Geometry check sheet. Reference: drawing and pictorial views, mm from the part's lowest x, y, z. A direction names the side the tool comes from. Give positions to 0.01 mm unless a question says otherwise; leave off trailing zeros. Loops run counter-clockwise (first coordinate to the right, second up) from the corner with the lowest first, then second, coordinate; pieces in that order, holes last. Notation, with made-up numbers: (32, 34.25) -> (85, 34.25) arc R33 cw to (85, 62.25) -> close; hole circle Ø7 at (-2, 23.5). An arc over 180 degrees is marked (long way). One line per item, written item: value. Start each with the question number.
(1) Gauge pin test, flat ends, axial feed: pin 1 Ø1.4 at (x, y) = (6.39, 19.11) entering from +Z; pin 2 Ø2 at (x, y) = (12.75, 3.75) entering from -Z; pin 3 Ø1.5 at (x, z) = (17, 2.5) entering from +Y. Record the tip position at first contact, or that the pin passes through.
(2) Sectioned sample at A-A, the plane y = 12.75. Record the cut outline in (x, z).
(3) Scan lines: line 1 along X through (y, z) = (6, 5.15); line 2 along Y through (x, z) = (12.75, 4.5); line 3 along Z through (x, y) = (10.5, 24). Record each from-to range of solid material in increasing order. Write a range as from..to.
(4) Tool access check on the marked faces 1 and 2. Record the directions out of +Z, -Z, +X, -X, +Y, -Y that give a thin tool (end or side, any length) a straight path to the whole face; none if there is none.
(5) Draft check along Y on the marked faces 3, 4 and 5. Enter one of: pulls with the +Y half, pulls with the -Y half, needs draft (parallel to the pull), parting line crosses it, or undercut.
(6) Sectioned sample at D-D, the plane x = 3.75. Record the cut outline in (y, z).
(7) Sectioned sample at C-C, the plane z = 1.85. Record the cut outline in (x, y), then the cut area to 3 significant figures.
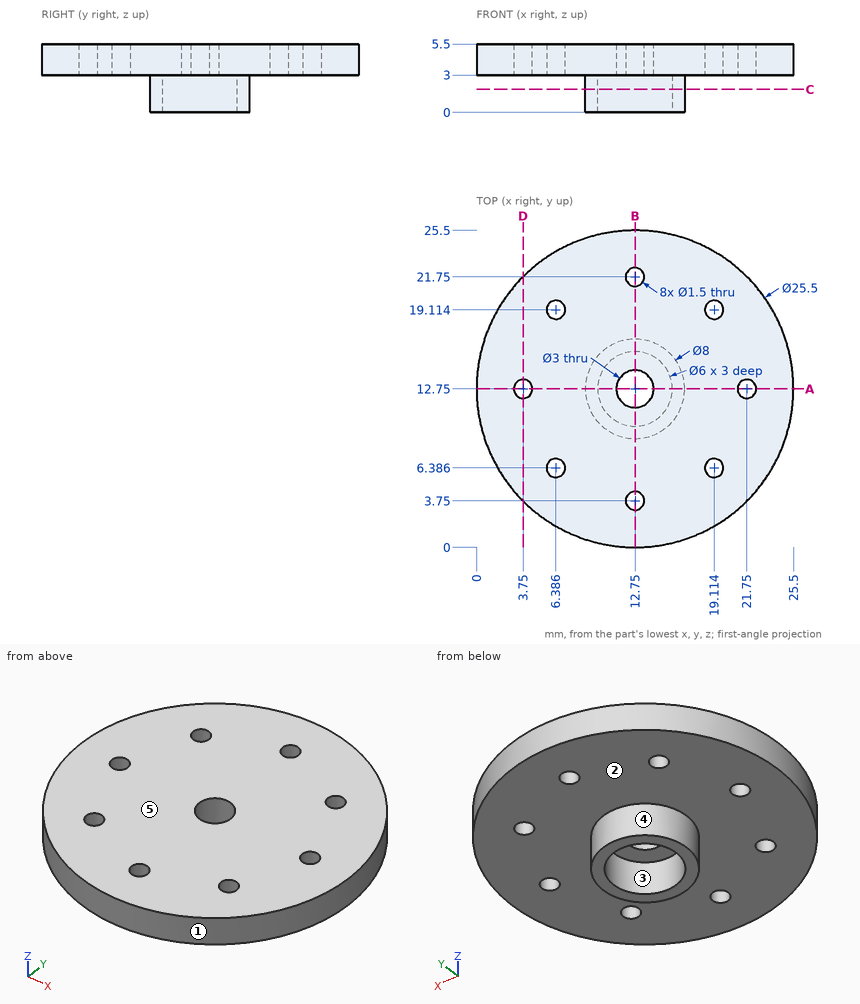
Calculated:
1. pin 1: passes through
1. pin 2: stops at z = 3
1. pin 3: stops at y = 24.95
2. outline: (0, 3) -> (3, 3) -> (3, 5.5) -> (0, 5.5) -> close; (4.5, 3) -> (8.75, 3) -> (8.75, 0) -> (9.75, 0) -> (9.75, 3) -> (11.25, 3) -> (11.25, 5.5) -> (4.5, 5.5) -> close; (14.25, 3) -> (15.75, 3) -> (15.75, 0) -> (16.75, 0) -> (16.75, 3) -> (21, 3) -> (21, 5.5) -> (14.25, 5.5) -> close; (22.5, 3) -> (25.5, 3) -> (25.5, 5.5) -> (22.5, 5.5) -> close
3. line 1: x = 1.93..5.74, 7.03..18.47, 19.76..23.57
3. line 2: y = 0..3, 4.5..11.25, 14.25..21, 22.5..25.5
3. line 3: z = 3..5.5
4. face 1: +Z, -Z
4. face 2: -Z
5. face 3: undercut
5. face 4: parting line crosses it
5. face 5: needs draft
6. outline: (3.72, 3) -> (12, 3) -> (12, 5.5) -> (3.72, 5.5) -> close; (13.5, 3) -> (21.78, 3) -> (21.78, 5.5) -> (13.5, 5.5) -> close
7. outline: circle Ø8 at (12.75, 12.75); hole circle Ø6 at (12.75, 12.75)
7. area: 22.0 mm2
